Geometry: final body of the model. Coordinates: model frame, mm. A direction names the side the tool comes from. Round coordinates to 2 decimals unless told otherwise and drop trailing zeros. Write each loop counter-clockwise with the first axis right and the second up, starting at its lowest first coordinate (ties: lowest second). Pieces come first, ordered by that corner, then holes. Notation, with made-up numbers: (69, 12.25) -> (87, 12.25) arc R22 ccw to (87, 38.25) -> close; hole circle Ø1 at (-31, -17). An arc over 180 degrees is marked (long way). One line per item, written item: value. Start each with the question number.
from build123d import *

# Parameters (mm, degrees)
ESQUISSE1_W             = 85
ESQUISSE1_H             = 40
ESQUISSE1_R             = 1.75
BOSS_EXTRU_1_DEPTH      = 2.5
ESQUISSE2_W             = 3
ESQUISSE2_H             = 17
BOSS_EXTRU_2_DEPTH      = 12
ESQUISSE3_R             = 1.75
ENL_V_MAT_EXTRU_1_DEPTH = 59
CONG_1_R                = 2.5


with BuildPart() as part:
    # Esquisse1 → Boss.-Extru.1 (new body)
    with BuildSketch(Plane.XY):
        with Locations((42.5, 20)):
            Rectangle(ESQUISSE1_W, ESQUISSE1_H)
        with Locations((23, 36.2)):
            Circle(ESQUISSE1_R, mode=Mode.SUBTRACT)
        with Locations((3.8, 3.8)):
            Circle(ESQUISSE1_R, mode=Mode.SUBTRACT)
        with Locations((81.2, 24)):
            Circle(ESQUISSE1_R, mode=Mode.SUBTRACT)
    extrude(amount=BOSS_EXTRU_1_DEPTH)

    # Esquisse2 → Boss.-Extru.2 (add)
    with BuildSketch(Plane(origin=(0, 0, 0), x_dir=(-1, 0, 0), z_dir=(0, 0, -1))):
        with Locations((-56.5, 20)):
            Rectangle(ESQUISSE2_W, ESQUISSE2_H)
    extrude(amount=BOSS_EXTRU_2_DEPTH)

    # Esquisse3 → Enlèv. mat.-Extru.1 (cut, through all)
    with BuildSketch(Plane(origin=(58, 0, 0), x_dir=(0, 0, -1), z_dir=(1, 0, 0))):
        with Locations((8.5, 24.25)):
            Circle(ESQUISSE3_R)
        with Locations((8.5, 15.75)):
            Circle(ESQUISSE3_R)
    extrude(amount=-ENL_V_MAT_EXTRU_1_DEPTH, mode=Mode.SUBTRACT)

    # Congé1
    cong_1_edges = [part.edges().sort_by_distance(p)[0] for p in [
        (56.5, 11.5, 0),
        (56.5, 28.5, 0),
        (56.5, 11.5, -12),
        (56.5, 28.5, -12),
    ]]
    fillet(cong_1_edges, radius=CONG_1_R)


solid = part.part
(1) Section query D-D (y = 20.5). Output: boundary loops of the cut face in (x, z), and give its area (4 significant figures).
(2) Section query A-A (y = 3.8). Output: boundary loops of the cut face in (x, z).
(3) Set-up query: faces 1 (the face through (55, 20, -6)), 2 (the face through (58, 20, -6)), 3 (the face through (57, 28.5, -6)). Return all of +Z, -Z, +X, -X, +Y, -Y with unobstructed straight access to the full face (end or side cutting, diameter ignored); none if empty.
(4) Line query: probe 1 along Y at (x, z) = (56.45, -8.5); probe 2 along Z at (x, y) = (55.5, 24); probe 3 along Y at (x, z) = (3.8, 1.05). Output: solid intervals per line, ascending.
(5) Pull-direction query (X, two-part tool) for faces 4 (the face through (85, 20, 1)), 5 (the face through (42, 40, 1)), 6 (the face through (80.972, 25.735, 1.232)); classes: pulls with the +X half, pulls with the -X half, needs draft (parallel to the pull), parting line crosses it, or undercut.
(6) Section query C-C (x = 23). Output: boundary loops of the cut face in (y, z).
(7) Pin query (flat end, axial travel): pin 1 (5.5 mm diameter, centred on y = 24.25, z = -8.5, fed in from +X); pin 2 (1 mm diameter, centred on y = 24.5, z = -2.5, fed in from -X); pin 3 (8 mm diameter, centred on x = 43.5, y = 13.5, fed in from -Z). Return the tip coordinate at first contact, or that it passes through.
(8) Section query B-B (z = -8.5). Output: boundary loops of the cut face in (x, y), and give its area (3 significant figures).
Results list:
1. outline: (0, 0) -> (55, 0) -> (55, -12) -> (58, -12) -> (58, 0) -> (85, 0) -> (85, 2.5) -> (0, 2.5) -> close
1. area: 248.5 mm^2
2. outline: (0, 0) -> (2.05, 0) -> (2.05, 2.5) -> (0, 2.5) -> close; (5.55, 0) -> (85, 0) -> (85, 2.5) -> (5.55, 2.5) -> close
3. face 1: -Z, -X, +Y, -Y
3. face 2: -Z, +X, +Y, -Y
3. face 3: -Z, +X, -X, +Y
4. probe 1: y = 11.5 to 14, 17.5 to 22.5, 26 to 28.5
4. probe 2: z = -12 to -10.23, -6.77 to 2.5
4. probe 3: y = 0 to 2.05, 5.55 to 40
5. face 4: pulls with the +X half
5. face 5: needs draft
5. face 6: undercut
6. outline: (0, 0) -> (34.45, 0) -> (34.45, 2.5) -> (0, 2.5) -> close; (37.95, 0) -> (40, 0) -> (40, 2.5) -> (37.95, 2.5) -> close
7. pin 1: stops at x = 58
7. pin 2: stops at x = 55
7. pin 3: stops at z = 0
8. outline: (55, 11.5) -> (58, 11.5) -> (58, 14) -> (55, 14) -> close; (55, 17.5) -> (58, 17.5) -> (58, 22.5) -> (55, 22.5) -> close; (55, 26) -> (58, 26) -> (58, 28.5) -> (55, 28.5) -> close
8. area: 30.0 mm^2
